For this review, take the finished solid that the model builds, in its own axes (mm). Coordinates: 2 decimals unless noted, no trailing zeros.
```python
from build123d import *

# Parameters (mm, degrees)
F1_DEPTH      = 7
F3_DEPTH      = 80
F3_DEPTH_BACK = 25
F4_COUNT      = 10


# Not quite as in the source:
# - an extrude ends at something that could not be found from the text; its depth is read off the source's solid


with BuildPart() as f1:
    # F0 (on Top) → F1 (new body)
    with BuildSketch(Plane.XY):
        with BuildLine():
            ThreePointArc((9.2862347639, 5.8962567709), (10.5628732456, 3.0701317233), (11, 0))
            ThreePointArc((11, 0), (9.4389817008, -5.6485063912), (5.1989773724, -9.6938451752))
            Line((5.1989773724, -9.6938451752), (17.4936950276, -9.6938451752))
            ThreePointArc((17.4936950276, -9.6938451752), (19.3632887257, -5.0063010021), (20, 0))
            ThreePointArc((20, 0), (19.9371690623, 1.5840737934), (19.7490710217, 3.1581947026))
            Line((19.7490710217, 3.1581947026), (12.9913196682, 5.5989294212))
            ThreePointArc((12.9913196682, 5.5989294212), (12.1549883134, 5.8213640414), (11.2928291783, 5.8962567709))
            Line((11.2928291783, 5.8962567709), (9.2862347639, 5.8962567709))
        make_face()
        with BuildLine():
            ThreePointArc((5.1989773724, -9.6938451752), (-10.6404023576, 2.7895945347), (9.2862347639, 5.8962567709))
            Line((9.2862347639, 5.8962567709), (11.2928291783, 5.8962567709))
            ThreePointArc((11.2928291783, 5.8962567709), (12.1549883134, 5.8213640414), (12.9913196682, 5.5989294212))
            Line((12.9913196682, 5.5989294212), (19.7490710217, 3.1581947026))
            ThreePointArc((19.7490710217, 3.1581947026), (-19.6989755573, 3.4569295616), (17.4936950276, -9.6938451752))
            Line((17.4936950276, -9.6938451752), (5.1989773724, -9.6938451752))
        make_face()
        with BuildLine():
            ThreePointArc((20, 0), (19.3632887257, -5.0063010021), (17.4936950276, -9.6938451752))
            Line((17.4936950276, -9.6938451752), (40.8740527928, -9.6938451752))
            add(Edge.make_bspline(
                [(34.0516753495, -2.0075566135), (35.8141325987, -2.7740908853), (39.3168982789, -4.2975263847), (40.357193967, -7.9026709732), (40.8740527928, -9.6938451752)],
                knots=[0, 0, 0, 0, 0.5031616186, 1, 1, 1, 1], degree=3))
            Line((34.0516753495, -2.0075566135), (19.7490710217, 3.1581947026))
            ThreePointArc((19.7490710217, 3.1581947026), (19.9371690623, 1.5840737934), (20, 0))
        make_face()
    extrude(amount=F1_DEPTH)

    # F2 (on Top) → F3 (cut, two sides)
    with BuildSketch(Plane.XY) as f3_sk:
        with BuildLine():
            ThreePointArc((24.097783491, -5.1900828257), (22.3410218592, -4.5133442837), (22.484831512, -2.6362440549))
            ThreePointArc((22.484831512, -2.6362440549), (21.2063665687, -4.2559181051), (20.7374691963, -6.2653836794))
            ThreePointArc((20.7374691963, -6.2653836794), (21.7064439422, -7.2920152577), (23.1120903045, -7.1614673361))
            ThreePointArc((23.1120903045, -7.1614673361), (28.3759705314, -5.094612778), (33.5514694452, -2.8154607862))
            ThreePointArc((33.5514694452, -2.8154607862), (28.7888988276, -3.8605353205), (24.097783491, -5.1900828257))
        make_face()
    extrude(amount=-F3_DEPTH, mode=Mode.SUBTRACT)
    extrude(f3_sk.sketch, amount=F3_DEPTH_BACK, mode=Mode.SUBTRACT)

    # F4: F1 ×10 about axis
    f4_axis = Axis((0, 0, 7), (0, 0, 1))


with BuildPart() as f1_1:
    add(f1.part)
    for i in range(1, F4_COUNT):
        add(f1.part.rotate(f4_axis, i * 360 / F4_COUNT))


solid = f1_1.part
```
1) Consider section A-A (y = 29.5). Count the separate pieces of the cut face and the enclosed holes in it, then the cut area to 3 significant figures.
2) Clearance check with flat-ended pins moving along their axes: P1, Ø4, axis at y = 0.5, z = 5, coming from the -X side; P2, Ø1, axis at x = 31, z = 1, coming from the -Y side; P3, Ø1, axis at x = -26.5, z = 4, coming from the -Y side. State where each tip first meets the part, or that it passes through.
3) For L1, parallel to X at y = 8.5, z = 1.75; L2, parallel to Y at x = -5.5, z = 2; L3, parallel to Y at x = -6, z = 2.25, list the stretches that pass through material, from the lowest coordinate up.
4) The part is to be moulded in two halves that separate along X. For faces 1 (the face through (-21.08, 20.07, 3.45)), 2 (the face through (27.36, 0.41, 3.45)), 3 (the face through (9, -9, 0)), say which applies: pulls with the +X half, pulls with the -X half, needs draft (parallel to the pull), parting line crosses it, or undercut.
Results:
1. separate pieces: 5
1. enclosed holes: 0
1. area: 147 mm2
2. P1: stops at x = -35.17
2. P2: stops at y = -9.69
2. P3: stops at y = -17.89
3. L1: x = -40.52 to -6.98, 6.98 to 19.78, 23.38 to 28.19
3. L2: y = -22.85 to -9.53, 9.53 to 29.01, 30.37 to 40.37
3. L3: y = -23.49 to -9.22, 9.22 to 29.83, 30.93 to 39.94
4. face 1: undercut
4. face 2: pulls with the +X half
4. face 3: needs draft
